Source: CAD feature listing. Evaluate the final solid. Frame: model axes, mm. Face numbers are marked on the shaded views. A direction names the side the tool comes from. Give positions to 0.01 mm unless a question says otherwise; leave off trailing zeros. Write each loop counter-clockwise with the first axis right and the second up, starting at its lowest first coordinate (ties: lowest second). Pieces come first, ordered by that corner, then holes. Notation, with made-up numbers: (81, 15) -> (113, 15) arc R29 cw to (113, 46) -> close; hole circle Ø1 at (37.5, -1.5). An arc over 180 degrees is marked (long way). Write item = value, one per line.
from build123d import *

# Parameters (mm, degrees)
SKETCH_R     = 4.58
PAD_DEPTH    = 1.55
SKETCH001_W  = 5
SKETCH001_H  = 5
PAD001_DEPTH = 1.6
SKETCH002_R  = 1.7
POCKET_DEPTH = 0.2
FILLET_R     = 0.1


with BuildPart() as part:
    # Sketch → Pad (new body)
    with BuildSketch(Plane.XY):
        Circle(SKETCH_R)
    extrude(amount=PAD_DEPTH)

    # Sketch001 (on Face3 of Pad) → Pad001 (join)
    with BuildSketch(Plane.XY.offset(1.55)):
        Rectangle(SKETCH001_W, SKETCH001_H)
    extrude(amount=PAD001_DEPTH)

    # Sketch002 (on Face8 of Pad001) → Pocket (cut)
    with BuildSketch(Plane.XY.offset(3.15)):
        Circle(SKETCH002_R)
    extrude(amount=-POCKET_DEPTH, mode=Mode.SUBTRACT)

    # Fillet
    fillet_edges = [part.edges().sort_by_distance(p)[0] for p in [
        (-4.58, 0, 0),
        (-4.58, 0, 1.55),
    ]]
    fillet(fillet_edges, radius=FILLET_R)


solid = part.part
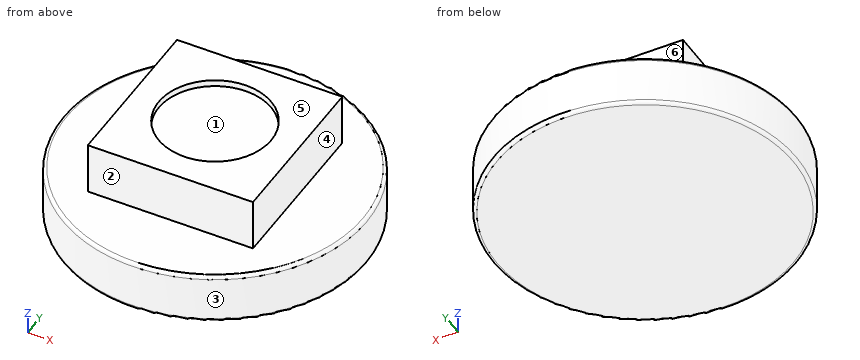
1) Access query for the marked faces 4, 5 and 6. Directions: +Z, -Z, +X, -X, +Y, -Y. A direction counts if a zero-diameter tool reaches every point of the face in a straight line with its end or side. Return the directions, or none.
Computed:
face_4 = +Z, +X, +Y, -Y
face_5 = +Z, +X, -X, +Y, -Y
face_6 = +Z, +X, -X, +Y
2) Cut plane D-D (z = 0.7). Return the cut outline in (x, y), then the cut area to 3 significant figures.
Computed:
outline = circle Ø9.16 at (0, 0)
area = 65.9 mm²
3) Contact query for flat-ended pins moving along their axis: pin 1 (1.8 mm diameter, centred on x = 1, z = 2, fed in from +Y); pin 2 (3 mm diameter, centred on x = 0, y = 0, fed in from +Z); pin 3 (1.8 mm diameter, centred on x = -1, z = 2.5, fed in from -Y). Output: stop coordinate, or through.
Computed:
pin_1 = 4.57
pin_2 = 2.95
pin_3 = -2.5
4) Draft query along Y for the marked faces 1, 2 and 3. Return one class per face: pulls with the +Y half, pulls with the -Y half, needs draft (parallel to the pull), parting line crosses it, or undercut.
Computed:
face_1 = undercut
face_2 = pulls with the -Y half
face_3 = parting line crosses it
5) Material intervals for L1, parallel to Y at x = 0, z = 3.05; L2, parallel to Z at x = 1.25, y = -2.75; L3, parallel to Z at x = -0.5, y = 1, sorted ascending.
Computed:
L1 = -2.5 to -1.7, 1.7 to 2.5
L2 = 0 to 1.55
L3 = 0 to 2.95
6) Cut plane C-C (z = 1.7). Return the cut outline in (x, y), then the cut area to 3 significant figures.
Computed:
outline = (-2.5, -2.5) -> (2.5, -2.5) -> (2.5, 2.5) -> (-2.5, 2.5) -> close
area = 25.0 mm²
7) Cut plane A-A (x = 0). Return the cut outline in (y, z).
Computed:
outline = (-4.58, 0.1) arc R0.1 ccw to (-4.48, 0) -> (4.48, 0) arc R0.1 ccw to (4.58, 0.1) -> (4.58, 1.45) arc R0.1 ccw to (4.48, 1.55) -> (2.5, 1.55) -> (2.5, 3.15) -> (1.7, 3.15) -> (1.7, 2.95) -> (-1.7, 2.95) -> (-1.7, 3.15) -> (-2.5, 3.15) -> (-2.5, 1.55) -> (-4.48, 1.55) arc R0.1 ccw to (-4.58, 1.45) -> close
